Could you check a few things on this model? Use its own coordinates, in mm. Face numbers are marked on the shaded views. A direction names the side the tool comes from. Round coordinates to 2 decimals unless told otherwise and drop trailing zeros. Loops run counter-clockwise (first coordinate to the right, second up) from the corner with the lowest first, then second, coordinate; pieces in that order, holes last. Notation, with made-up numbers: (24.25, -4.5) - (72.25, -4.5) arc R27 cw to (72.25, 27.5) - close; hole circle Ø2 at (8.25, -36.5). An arc over 180 degrees is marked (long way). Answer as CSV lines item,"result". Start each with the question number.
1) Suppose I cut it at C-C, the plane x = -3. Write out the boundary of the cut face in (y, z).
2) Suppose I cut it at D-D, the plane z = 18.25. Write out the boundary of the cut face in (x, y) (3 decimals).
3) Suppose I cut it at B-B, the plane z = 10.75. Count the separate pieces of the cut face and the enclosed holes in it, then the cut area to 3 significant figures.
4) Which directions (+Z, -Z, +X, -X, +Y, -Y) give clear straight access to the entire face, cutting with the end or side of a thin tool? Please do the marked faces 4 and 5.
5) I'm going to push flat-ended pins straight in: pin 1 Ø4.5 at (x, y) = (-2.42, 18.35) entering from +Z; pin 2 Ø2 at (x, z) = (-3.5, 9.5) entering from -Y; pin 3 Ø5 at (x, z) = (7, 22) entering from +Y; pin 4 Ø1.5 at (y, z) = (-6, 6) entering from -X. Where does each tip first touch, or does it pass through?
6) We'd pull the mould along X, two halves only. Please class the marked faces 1, 2 and 3: pulls with the +X half, pulls with the -X half, needs draft (parallel to the pull), parting line crosses it, or undercut.
7) Please list where these lines run through material, in increasing order: line 1 along Y through (x, z) = (0, 11.25) (1 decimal); line 2 along X through (y, z) = (1, 11); line 3 along Z through (x, y) = (12, -2).
8) Suppose I cut it at A-A, the plane y = -2. Write out the boundary of the cut face in (x, z), then the cut area to 3 significant figures.
```python
from build123d import *

# Parameters (mm, degrees)
SKETCH1_W                = 23.025
SKETCH1_H                = 15
SKETCH2_R                = 22.575
BOSS_EXTRUDE1_DEPTH      = 13
HOLE1_D                  = 20
HOLE1_CBORE_D            = 28
HOLE1_CBORE_DEPTH        = 27
M2_CLEARANCE_HOLE1_D     = 2.459
M2_CLEARANCE_HOLE1_DEPTH = 14.999999999
M2_CLEARANCE_HOLE1_TIP   = 0.738758131
SKETCH7_R                = 1.8288
CUT_EXTRUDE1_DEPTH       = 11.557
SKETCH8_R                = 2.032
CUT_EXTRUDE2_DEPTH       = 1.016


with BuildPart() as part:
    # Sketch1 → Revolve1 (revolve)
    with BuildSketch(Plane(origin=(0, 0, 0), x_dir=(1, 0, 0), z_dir=(0, 1, 0))):
        with Locations((11.5125, -20.5)):
            Rectangle(SKETCH1_W, SKETCH1_H)
    revolve(axis=Axis((0, 0, 13), (0, 0, 1)))

    # Sketch2 → Boss-Extrude1 (add)
    with BuildSketch(Plane(origin=(0, 0, 13), x_dir=(-1, 0, 0), z_dir=(0, 0, -1))):
        with Locations(Location((0, 0, 0), (0, 0, 180))):
            Circle(SKETCH2_R)
    extrude(amount=BOSS_EXTRUDE1_DEPTH)

    # Hole1 (through all)
    with Locations(Plane.XY.offset(28)):
        with Locations((0, 0)):
            CounterBoreHole(HOLE1_D / 2, HOLE1_CBORE_D / 2, HOLE1_CBORE_DEPTH)

    # M2 Clearance Hole1
    with Locations(Plane(origin=(0, 0, 0), x_dir=(-1, 0, 0), z_dir=(0, 0, -1))):
        with Locations((0, 17.5), (-17.5, 0), (0, -17.5), (17.5, 0)):
            Hole(M2_CLEARANCE_HOLE1_D / 2, depth=M2_CLEARANCE_HOLE1_DEPTH)
            with Locations((0, 0, -(M2_CLEARANCE_HOLE1_DEPTH + M2_CLEARANCE_HOLE1_TIP / 2))):  # 118° drill point
                Cone(0, M2_CLEARANCE_HOLE1_D / 2, M2_CLEARANCE_HOLE1_TIP, mode=Mode.SUBTRACT)

    # Sketch7 → Cut-Extrude1 (cut)
    with BuildSketch(Plane.XY.offset(28)):
        with Locations((-2.416366133, 18.354122996)):
            Circle(SKETCH7_R)
        with Locations((-7.084427042, 17.103319846)):
            Circle(SKETCH7_R)
        with Locations((-11.269695955, 14.686953712)):
            Circle(SKETCH7_R)
        with Locations(Location((11.269695955, 14.686953712, 0), (0, 0, 180))):
            Circle(SKETCH7_R)
        with Locations(Location((7.084427042, 17.103319846, 0), (0, 0, 180))):
            Circle(SKETCH7_R)
        with Locations(Location((2.416366133, 18.354122996, 0), (0, 0, 180))):
            Circle(SKETCH7_R)
    extrude(amount=-CUT_EXTRUDE1_DEPTH, mode=Mode.SUBTRACT)

    # Sketch8 → Cut-Extrude2 (cut)
    with BuildSketch(Plane.XY.offset(28)):
        with Locations((-11.269695955, 14.686953712)):
            Circle(SKETCH8_R)
        with Locations((-7.084427042, 17.103319846)):
            Circle(SKETCH8_R)
        with Locations((-2.416366133, 18.354122996)):
            Circle(SKETCH8_R)
        with Locations((2.416366133, 18.354122996)):
            Circle(SKETCH8_R)
        with Locations((7.084427042, 17.103319846)):
            Circle(SKETCH8_R)
        with Locations((11.269695955, 14.686953712)):
            Circle(SKETCH8_R)
    extrude(amount=-CUT_EXTRUDE2_DEPTH, mode=Mode.SUBTRACT)


solid = part.part
```
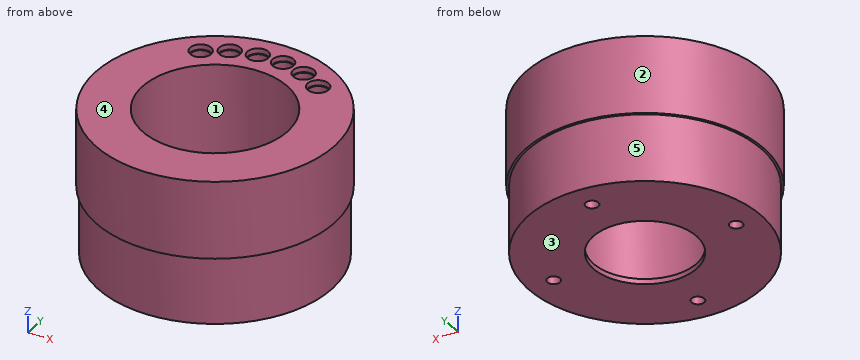
Filled sheet:
1,outline,"(-22.83, 13) - (-22.37, 13) - (-22.37, 0) - (-9.54, 0) - (-9.54, 1) - (-13.67, 1) - (-13.67, 28) - (-22.83, 28) - close; (9.54, 0) - (22.37, 0) - (22.37, 13) - (22.83, 13) - (22.83, 28) - (20.3, 28) - (20.3, 26.98) - (20.09, 26.98) - (20.09, 16.44) - (16.62, 16.44) - (16.62, 26.98) - (16.41, 26.98) - (16.41, 28) - (13.67, 28) - (13.67, 1) - (9.54, 1) - close"
2,outline,"circle Ø46.05 at (0, 0); hole circle Ø28 at (0, 0); hole circle Ø3.658 at (-11.27, 14.687); hole circle Ø3.658 at (-7.084, 17.103); hole circle Ø3.658 at (-2.416, 18.354); hole circle Ø3.658 at (2.416, 18.354); hole circle Ø3.658 at (7.084, 17.103); hole circle Ø3.658 at (11.27, 14.687)"
3,separate pieces,"1"
3,enclosed holes,"5"
3,area,"966 mm²"
4,face 4,"+Z, +X, -X, +Y, -Y"
4,face 5,"-Z"
5,pin 1,"z = 28"
5,pin 2,"y = -22.44"
5,pin 3,"y = 22.58"
5,pin 4,"x = -21.96"
6,face 1,"undercut"
6,face 2,"parting line crosses it"
6,face 3,"needs draft"
7,line 1,"-22.6 to -18.7, -16.3 to -14, 14 to 16.3, 18.7 to 22.6"
7,line 2,"-22.55 to -18.22, -16.78 to -13.96, 13.96 to 16.78, 18.22 to 22.55"
7,line 3,"0 to 1"
8,outline,"(-22.94, 13) - (-22.49, 13) - (-22.49, 0) - (-9.8, 0) - (-9.8, 1) - (-13.86, 1) - (-13.86, 28) - (-22.94, 28) - close; (9.8, 0) - (22.49, 0) - (22.49, 13) - (22.94, 13) - (22.94, 28) - (13.86, 28) - (13.86, 1) - (9.8, 1) - close"
8,area,"505 mm²"
